Verification items for the finished model (mm, model axes). A direction names the side the tool comes from. Coordinates: 2 decimals unless noted, no trailing zeros. Write each loop counter-clockwise with the first axis right and the second up, starting at its lowest first coordinate (ties: lowest second). Pieces come first, ordered by that corner, then holes. Notation, with made-up numbers: (39.25, 32) -> (57.25, 32) arc R18 ccw to (57.25, 57) -> close; hole circle Ø6 at (-21, 41). An arc over 180 degrees is marked (long way). Answer in a Markdown table with one row per item.
Autodesk Inventor part; units mm, degrees
ref_plane "YZ Plane" through (0, 0, 0) normal (1, 0, 0) x (0, 1, 0)
ref_plane "XZ Plane" through (0, 0, 0) normal (0, 1, 0) x (-1, 0, 0)
ref_plane "XY Plane" through (0, 0, 0) normal (0, 0, 1) x (1, 0, 0)
sketch "Sketch1" plane through (0, 0, 0) normal (0, 1, 0) x (-1, 0, 0)
  line L0 (0, 4) -> (-20, 4)
  line L1 (-20, 4) -> (-20, -4)
  line L2 (-20, -4) -> (0, -4)
  circle A0 centre (-20, 0) radius 4
  circle A1 centre (-20, 0) radius 2.5
  line L3 (-20, -4) -> (-30, -4)
  line L4 (-30, -4) -> (-30, 4)
  line L5 (-30, 4) -> (-20, 4)
  line L6 (-20, 4) -> (-20, -4)
  circle A2 centre (4, 0) radius 4
  circle A3 centre (4, 0) radius 2.5
  line L7 (0, 4) -> (4, 4)
  line L8 (4, -4) -> (0, -4)
  point P0 (-20, -2.5)
  point P1 (-20, 2.5)
  dimension "d32" = 20
  dimension "d34" = 5
  dimension "d47" = 10
  dimension "d48" = 5
extrude "Extrusion1" add sketch "Sketch1" along normal blind 2 contours L7 A2 L8 L2 A0 L0 | A0 L1 A1 | L1 A1 A0 | A0 L3 L4 L5 | A2
thread "Thread2"
sketch "Sketch4" plane through (0, 0, 0) normal (0, -1, 0) x (1, 0, 0)
  circle A0 centre (10, 0) radius 1.5
  point P0 (0, 0)
  dimension "d46" = 3
extrude "Extrusion5" add sketch "Sketch4" along normal blind 5
thread "Thread3"
properties part number "link"
1. Section check A-A, the plane z = 0. Record the boundary of the cut face in (x, y), plus the area to 3 significant figures.
Geometry says:
| item | result |
|---|---|
| outline | (-8, 0) -> (-6.5, 0) -> (-6.5, 2) -> (-8, 2) -> close; (-1.5, 0) -> (8.5, 0) -> (8.5, -5) -> (11.5, -5) -> (11.5, 0) -> (17.5, 0) -> (17.5, 2) -> (-1.5, 2) -> close; (22.5, 0) -> (30, 0) -> (30, 2) -> (22.5, 2) -> close |
| area | 71.0 mm^2 |
2. Section check D-D, the plane z = 2. Record the boundary of the cut face in (x, y), plus the area to 3 significant figures.
Geometry says:
| item | result |
|---|---|
| outline | (-7.46, 0) -> (-5.5, 0) -> (-5.5, 2) -> (-7.46, 2) -> close; (-2.5, 0) -> (18.5, 0) -> (18.5, 2) -> (-2.5, 2) -> close; (21.5, 0) -> (30, 0) -> (30, 2) -> (21.5, 2) -> close |
| area | 62.9 mm^2 |
3. Thickness scan on line 1 (Z direction, x = 20, y = 1.4); line 2 (Y direction, x = 4.5, z = -3); line 3 (X direction, y = -2, z = -0.5). Record the ranges inside material, lowest first. Write a range as from..to.
Geometry says:
| item | result |
|---|---|
| line 1 | -4..-2.5, 2.5..4 |
| line 2 | 0..2 |
| line 3 | 8.59..11.41 |
4. Section check C-C, the plane x = 10. Record the boundary of the cut face in (y, z), plus the area to 3 significant figures.
Geometry says:
| item | result |
|---|---|
| outline | (-5, -1.5) -> (0, -1.5) -> (0, -4) -> (2, -4) -> (2, 4) -> (0, 4) -> (0, 1.5) -> (-5, 1.5) -> close |
| area | 31.0 mm^2 |
5. Depth check by flat-ended pin: P1, Ø3, axis at y = -3.5, z = 1.5, coming from the -X side; P2, Ø4, axis at x = 17.5, z = -0.5, coming from the -Y side; P3, Ø1, axis at x = 8.5, z = 0.5, coming from the -Y side; P4, Ø4.5, axis at x = 20, z = 0, coming from the +Y side. Enter the tip coordinate at first touch or a pass-through.
Geometry says:
| item | result |
|---|---|
| P1 | x = 8.5 |
| P2 | y = 0 |
| P3 | y = -5 |
| P4 | through |
6. Mould release check, pull along X, two halves, no side actions. Record for faces 3 (the flat face through (30, 1, 0)), 4 (the cylindrical face through (22.5, 1, -0.1)), 5 (the flat face through (11, 0, 2)), 6 (the cylindrical face through (-8, 1, 0)): released by +X, released by -X, zero draft, split by the parting line, or undercut.
Geometry says:
| item | result |
|---|---|
| face 3 | released by +X |
| face 4 | undercut |
| face 5 | zero draft |
| face 6 | released by -X |
7. Tool access check on faces 1 (the cylindrical face through (-6.385, 0.986, -0.751)), 2 (the cylindrical face through (8.5, -2.46, -0.07)). Record the directions out of +Z, -Z, +X, -X, +Y, -Y that give a thin tool (end or side, any length) a straight path to the whole face; none if there is none.
Geometry says:
| item | result |
|---|---|
| face 1 | +Y, -Y |
| face 2 | -Y |
8. Section check B-B, the plane y = 0.5. Record the boundary of the cut face in (x, z).
Geometry says:
| item | result |
|---|---|
| outline | (-4, -4) -> (30, -4) -> (30, 4) -> (-4, 4) arc R4 ccw to start; hole circle Ø5 at (-4, 0); hole circle Ø5 at (20, 0) |
